```python
from build123d import *

# Parameters (mm, degrees)
CROQUIS1_R              = 1.475
SALIENTE_EXTRUIR1_DEPTH = 108
CHAFL_N1_SIZE           = 0.5
CHAFL_N1_SIZE2          = 0.288675135
CHAFL_N2_SIZE           = 0.5


with BuildPart() as part:
    # Croquis1 → Saliente-Extruir1 (new body)
    with BuildSketch(Plane(origin=(0, 0, 0), x_dir=(0, 0, -1), z_dir=(1, 0, 0))):
        Circle(CROQUIS1_R)
    extrude(amount=SALIENTE_EXTRUIR1_DEPTH)

    # Chaflán1
    chafl_n1_edges = [part.edges().sort_by_distance(p)[0] for p in [
        (108, 0, 1.475),
    ]]
    chafl_n1_side = [part.faces().sort_by_distance(p)[0] for p in [
        (54, 0, 1.475),
    ]]
    chamfer(chafl_n1_edges, length=CHAFL_N1_SIZE, length2=CHAFL_N1_SIZE2, reference=chafl_n1_side[0])

    # Chaflán2
    chafl_n2_edges = [part.edges().sort_by_distance(p)[0] for p in [
        (0, 0, 1.475),
    ]]
    chamfer(chafl_n2_edges, length=CHAFL_N2_SIZE)


solid = part.part
```
Check sheet for the modelled part. Datum: model origin and axes. Units: mm. Coordinates: 2 decimals unless noted, no trailing zeros. Loops run counter-clockwise (first coordinate to the right, second up) from the corner with the lowest first, then second, coordinate; pieces in that order, holes last.
1) Gauge pin test, flat end, axial feed: pin 1 (1 mm diameter, centred on x = 21, y = 1, fed in from -Z). Record the tip position at first contact, or that the pin passes through.
2) Material ranges on probe 1 along Z at (x, y) = (29, 1.1); probe 2 along Y at (x, z) = (38, 0.1), recorded low to high.
3) Sectioned sample at A-A (x = 13). Record the boundary of the cut face in (y, z) (3 decimals).
Check sheet entries:
1. pin 1: stops at z = -1.39
2. probe 1: z = -0.98 to 0.98
2. probe 2: y = -1.47 to 1.47
3. outline: circle Ø2.95 at (0, 0)
